Verification items for the finished model (mm, model axes). A direction names the side the tool comes from. Give positions to 0.01 mm unless a question says otherwise; leave off trailing zeros. Order: outer loops, then holes, each group sorted by start corner. A loop starts at its lowest first (then second) coordinate and runs counter-clockwise, first axis right, second up. Notation, with made-up numbers: (27, 39) - (34, 39) arc R22 ccw to (34, 45) - close; hole circle Ø7 at (9, 44.5). An arc over 180 degrees is marked (long way). Answer as a JSON object with one key per item and string values. Group by question number.
(1) Depth check by flat-ended pin: pin 1 Ø2 at (y, z) = (18.5, 29) entering from +X; pin 2 Ø1 at (x, y) = (-52, 45) entering from -Z. Enter the tip coordinate at first touch or a pass-through.
(2) Section check D-D (z = 11). Record the boundary of the cut face in (x, y).
(3) Section check A-A (x = -28.5). Record the boundary of the cut face in (y, z), then the cut area to 3 significant figures.
(4) Mould release check, pull along Y, two halves, no side actions. Record for faces 4 (the face through (-53, 74, 15)), 5 (the face through (-104, 36, 15)), 6 (the face through (-53, 0, 15)), 7 (the face through (-62, 37, 28)): +Y half, -Y half, draft (parallel to the pull), parting line (faces both ways), or undercut.
(5) Section check C-C (x = -40). Record the boundary of the cut face in (y, z).
(6) Thickness scan on line 1 (Y direction, x = -28, z = 28.75); line 2 (X direction, y = 65, z = 22); line 3 (Y direction, x = -23, z = 11). Record the ranges inside material, lowest first.
(7) Access from +Z, -Z, +X, -X, +Y, -Y to the whole of each face (thin tool, end or side, straight path). Record for faces 1 (the face through (-102, 37, 15)), 2 (the face through (-100, 42, 29)), 3 (the face through (0, 36, 15)).
(8) Section check B-B (y = 61.5). Record the boundary of the cut face in (x, z), then the cut area to 3 significant figures.
```python
from build123d import *

# Parameters (mm, degrees)
SKETCH1_W           = 104
SKETCH1_H           = 74
SKETCH1_W_2         = 5
SKETCH1_H_2         = 40
SKETCH1_W_3         = 40
SKETCH1_W_4         = 30
SKETCH1_H_3         = 25
BOSS_EXTRUDE1_DEPTH = 30
SKETCH2_W           = 100
SKETCH2_H           = 70
CUT_EXTRUDE1_DEPTH  = 28


with BuildPart() as part:
    # Sketch1 → Boss-Extrude1 (new body)
    with BuildSketch(Plane.XY):
        with Locations((-52, 37)):
            Rectangle(SKETCH1_W, SKETCH1_H)
        with Locations((-99.5, 22)):
            Rectangle(SKETCH1_W_2, SKETCH1_H_2, mode=Mode.SUBTRACT)
        with Locations((-22, 22)):
            Rectangle(SKETCH1_W_3, SKETCH1_H_2, mode=Mode.SUBTRACT)
        with Locations((-17, 59.5)):
            Rectangle(SKETCH1_W_4, SKETCH1_H_3, mode=Mode.SUBTRACT)
    extrude(amount=BOSS_EXTRUDE1_DEPTH)

    # Sketch2 → Cut-Extrude1 (cut)
    with BuildSketch(Plane(origin=(0, 0, 0), x_dir=(-1, 0, 0), z_dir=(0, 0, -1))):
        with Locations((52, 37)):
            Rectangle(SKETCH2_W, SKETCH2_H)
    extrude(amount=-CUT_EXTRUDE1_DEPTH, mode=Mode.SUBTRACT)


solid = part.part
```
Solutions:
{
 "1": {"pin 1": "stops at x = 0", "pin 2": "stops at z = 28"},
 "2": {"outline": "(-104, 0) - (0, 0) - (0, 74) - (-104, 74) - close; hole (-102, 2) - (-2, 2) - (-2, 72) - (-102, 72) - close"},
 "3": {"outline": "(0, 0) - (2, 0) - (2, 30) - (0, 30) - close; (42, 28) - (47, 28) - (47, 30) - (42, 30) - close; (72, 0) - (74, 0) - (74, 30) - (72, 30) - close", "area": "130 mm2"},
 "4": {"face 4": "+Y half", "face 5": "draft", "face 6": "-Y half", "face 7": "undercut"},
 "5": {"outline": "(0, 0) - (2, 0) - (2, 30) - (0, 30) - close; (42, 28) - (72, 28) - (72, 0) - (74, 0) - (74, 30) - (42, 30) - close"},
 "6": {"line 1": "y = 0 to 2, 42 to 47, 72 to 74", "line 2": "x = -104 to -102, -2 to 0", "line 3": "y = 0 to 2, 72 to 74"},
 "7": {"face 1": "-Z", "face 2": "+Z, -Z", "face 3": "+Z, -Z, +X, +Y, -Y"},
 "8": {"outline": "(-104, 0) - (-102, 0) - (-102, 28) - (-32, 28) - (-32, 30) - (-104, 30) - close; (-2, 0) - (0, 0) - (0, 30) - (-2, 30) - close", "area": "260 mm2"}
}
